Design review of the part built by this model. Coordinates are the model's own, in mm. A direction names the side the tool comes from. Coordinates: 2 decimals unless noted, no trailing zeros. Write each loop counter-clockwise with the first axis right and the second up, starting at its lowest first coordinate (ties: lowest second). Pieces come first, ordered by that corner, then holes. Notation, with made-up numbers: (-11, 18.25) - (-3, 18.25) arc R25 cw to (-3, 51.25) - close; hole circle Ø1 at (22.25, 86.25). An arc over 180 degrees is marked (long way). Answer as CSV lines item,"result". Start each with the question number.
Q1. We need section B-B (x = 40.5). Write out the cut boundary in (y, z), plus the area to 3 significant figures.
Q2. We need section D-D (z = 159). Write out the cut boundary in (x, y), plus the area to 3 significant figures.
Q3. We need section C-C (z = 23.5). Write out the cut boundary in (x, y), plus the area to 3 significant figures.
Q4. Clearance check with flat-ended pins moving along their axes: pin 1 (7 mm diameter, centred on x = -85.5, y = 72.5, fed in from +Z); pin 2 (5 mm diameter, centred on x = -83, y = -80.5, fed in from +Z); pin 3 (12 mm diameter, centred on x = 91, z = 99, fed in from +Y). State where each tip first meets the part, or that it passes through.
Q5. We need section A-A (y = -21.5). Write out the cut boundary in (x, z), plus the area to 3 significant figures.
Q6. Mouldability with a two-part tool opening along X and no side actions: class faces 4 (the face through (6.51, 76.54, 100.18)), 5 (the face through (5, -148.059, -6)), 6 (the face through (124.492, -26, -6)) as pulls with the +X half, pulls with the -X half, needs draft (parallel to the pull), parting line crosses it, or undercut.
Q7. For line 1 along Z through (x, y) = (-76, 15), list the stretches that pass through material, from the lowest coordinate up. Write a range as [from, to].
Q8. Machinability: for faces 1 (the face through (-85.92, 76.527, 75.133)), 2 (the face through (-86, 73, 152.4)), 3 (the face through (99, 73, 152.4)), which of the approach directions +Z, -Z, +X, -X, +Y, -Y give a long, thin tool a straight path to every point of the face, cutting with its end or side? Answer none if there is none.
from build123d import *

# Parameters (mm, degrees)
F0_W     = 235.324252
F0_H     = 247.140977
F1_DEPTH = 12.7
F2_R     = 3.200051
F3_DEPTH = 152.4
F4_R     = 3.156732
F5_DEPTH = 152.4
F6_R     = 3.21323
F7_DEPTH = 203.2


with BuildPart() as f1:
    # F0 (on Top) → F1 (new body)
    with BuildSketch(Plane.XY):
        with Locations((6.829398, -24.4885)):
            Rectangle(F0_W, F0_H)
    extrude(amount=-F1_DEPTH)

    # F2 (on face) → F3 (join)
    with BuildSketch(Plane.XY):
        with Locations((-85.502937, 73.354565)):
            Circle(F2_R)
    extrude(amount=F3_DEPTH)

    # F4 (on face) → F5 (join)
    with BuildSketch(Plane.XY):
        with Locations((99.039346, 73.238835)):
            Circle(F4_R)
    extrude(amount=F5_DEPTH)

    # F6 (on face) → F7 (join)
    with BuildSketch(Plane.XY):
        with Locations((6.923744, 73.353745)):
            Circle(F6_R)
    extrude(amount=F7_DEPTH)


solid = f1.part
Results list:
1,outline,"(-148.06, -12.7) - (99.08, -12.7) - (99.08, 0) - (-148.06, 0) - close"
1,area,"3,140 mm2"
2,outline,"circle Ø6.43 at (6.92, 73.35)"
2,area,"32.4 mm2"
3,outline,"circle Ø6.4 at (-85.5, 73.35); circle Ø6.43 at (6.92, 73.35); circle Ø6.31 at (99.04, 73.24)"
3,area,"95.9 mm2"
4,pin 1,"stops at z = 152.4"
4,pin 2,"stops at z = 0"
4,pin 3,"stops at y = 75.65"
5,outline,"(-110.83, -12.7) - (124.49, -12.7) - (124.49, 0) - (-110.83, 0) - close"
5,area,"2,990 mm2"
6,face 4,"undercut"
6,face 5,"needs draft"
6,face 6,"pulls with the +X half"
7,line 1,"z = [-12.7, 0]"
8,face 1,"+Z"
8,face 2,"+Z, -X, +Y, -Y"
8,face 3,"+Z, +X, +Y, -Y"
